from build123d import *

# Parameters (mm, degrees)
BOSS_EXTRUDE1_DEPTH = 12.7
FILLET2_R           = 2.54
SKETCH2_R           = 3.175
CUT_EXTRUDE1_DEPTH  = 12.7


with BuildPart() as part:
    # Sketch1 → Boss-Extrude1 (new body)
    with BuildSketch(Plane.XY):
        with BuildLine():
            ThreePointArc((31.750000111, -25.4), (6.35, -1.11e-07), (31.749999889, 25.4))
            Line((31.749999889, 25.4), (-63.5, 25.4))
            Line((-63.5, 25.4), (-63.5, -25.4))
            Line((-63.5, -25.4), (31.750000111, -25.4))
        make_face()
        with BuildLine():
            ThreePointArc((49.97081502, -7.62), (12, 0), (49.97081502, 7.62))
            Line((49.97081502, 7.62), (55.980055716, 7.62))
            ThreePointArc((55.980055716, 7.62), (46.776842604, 20.478134714), (31.749999889, 25.4))
            ThreePointArc((31.749999889, 25.4), (6.35, -1.11e-07), (31.750000111, -25.4))
            ThreePointArc((31.750000111, -25.4), (46.776842694, -20.478134648), (55.980055716, -7.62))
            Line((55.980055716, -7.62), (49.97081502, -7.62))
        make_face()
        with BuildLine():
            ThreePointArc((49.97081502, 7.62), (50.823284356, 5.125653506), (51.335987338, 2.54))
            Line((51.335987338, 2.54), (57.022680903, 2.54))
            ThreePointArc((57.022680903, 2.54), (56.631355132, 5.106678649), (55.980055716, 7.62))
            Line((55.980055716, 7.62), (49.97081502, 7.62))
        make_face()
        with BuildLine():
            ThreePointArc((55.980055716, 7.62), (56.631355132, 5.106678649), (57.022680903, 2.54))
            Line((57.022680903, 2.54), (63.5, 2.54))
            Line((63.5, 2.54), (63.5, 7.62))
            Line((63.5, 7.62), (55.980055716, 7.62))
        make_face()
        with BuildLine():
            Line((57.022680903, -2.54), (51.335987338, -2.54))
            ThreePointArc((51.335987338, -2.54), (50.823284356, -5.125653506), (49.97081502, -7.62))
            Line((49.97081502, -7.62), (55.980055716, -7.62))
            ThreePointArc((55.980055716, -7.62), (56.631355132, -5.106678649), (57.022680903, -2.54))
        make_face()
        with BuildLine():
            Line((63.5, -2.54), (57.022680903, -2.54))
            ThreePointArc((57.022680903, -2.54), (56.631355132, -5.106678649), (55.980055716, -7.62))
            Line((55.980055716, -7.62), (63.5, -7.62))
            Line((63.5, -7.62), (63.5, -2.54))
        make_face()
        with BuildLine():
            Line((63.5, -7.62), (55.980055716, -7.62))
            ThreePointArc((55.980055716, -7.62), (46.776842694, -20.478134648), (31.750000111, -25.4))
            Line((31.750000111, -25.4), (63.5, -25.4))
            Line((63.5, -25.4), (63.5, -7.62))
        make_face()
    extrude(amount=BOSS_EXTRUDE1_DEPTH)

    # Fillet2
    fillet2_edges = [part.edges().sort_by_distance(p)[0] for p in [
        (51.335987338, 2.54, 6.35),
        (51.335987338, -2.54, 6.35),
    ]]
    fillet(fillet2_edges, radius=FILLET2_R)

    # Sketch2 → Cut-Extrude1 (cut)
    with BuildSketch(Plane.XY.offset(12.7)):
        with Locations((-50.8, -9.525)):
            Circle(SKETCH2_R)
        with Locations((-41.819743879, -0.544743879)):
            Circle(SKETCH2_R)
        with Locations((-32.839487758, 8.435512242)):
            Circle(SKETCH2_R)
        with Locations((-41.148, -9.525)):
            Circle(SKETCH2_R)
        with Locations((-32.167743879, -0.544743879)):
            Circle(SKETCH2_R)
        with Locations((-23.187487758, 8.435512242)):
            Circle(SKETCH2_R)
        with Locations((-31.496, -9.525)):
            Circle(SKETCH2_R)
        with Locations((-22.515743879, -0.544743879)):
            Circle(SKETCH2_R)
        with Locations((-13.535487758, 8.435512242)):
            Circle(SKETCH2_R)
        with Locations((-21.844, -9.525)):
            Circle(SKETCH2_R)
        with Locations((-12.863743879, -0.544743879)):
            Circle(SKETCH2_R)
        with Locations((-3.883487758, 8.435512242)):
            Circle(SKETCH2_R)
    extrude(amount=-CUT_EXTRUDE1_DEPTH, mode=Mode.SUBTRACT)


solid = part.part
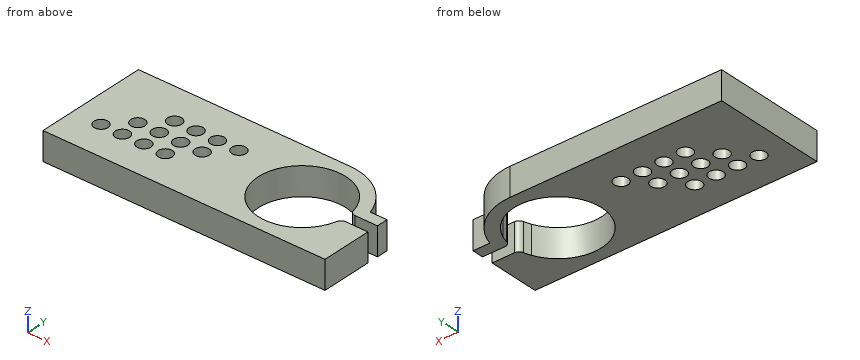
Build history of the part. All positions in model axes, mm. Give positions to 0.01 mm unless a question says otherwise; leave off trailing zeros. Write each loop counter-clockwise with the first axis right and the second up, starting at its lowest first coordinate (ties: lowest second). Pieces come first, ordered by that corner, then holes. Notation, with made-up numbers: (-5.5, 3.5) - (37.5, 3.5) arc R15 cw to (37.5, 9.5) - close; hole circle Ø10 at (78.25, 52). An arc over 180 degrees is marked (long way). Use one line per item in the form item = value. Start each with the question number.
1. Band-saw the part on B-B on y = 10. Write the cut outline in (x, z).
2. Band-saw the part on C-C on z = 10.75. Count the separate pieces of the cut face and the enclosed holes in it, plus the area to 3 significant figures.
3. Band-saw the part on D-D on x = -22.5. Write the cut outline in (y, z).
4. Probe line 1 (Y direction, x = 57, z = 10.5); line 2 (X direction, y = -7.5, z = 12); line 3 (X direction, y = 9, z = 4.5). List the from-to ranges inside material, lowest first. Write a range as [from, to].
5. Band-saw the part on A-A on x = -50.8. Write the cut outline in (y, z), plus the area to 3 significant figures.
6. Drop flat-ended pins along their axis: pin 1 Ø5 at (y, z) = (11.5, 8) entering from +X; pin 2 Ø4 at (x, z) = (60.5, 8) entering from +Y. Give the stop position or say it passes through.
Conclusion:
q1.outline = (-63.5, 0) - (-35.6, 0) - (-35.6, 12.7) - (-63.5, 12.7) - close; (-30.08, 0) - (-25.95, 0) - (-25.95, 12.7) - (-30.08, 12.7) - close; (-20.42, 0) - (-16.3, 0) - (-16.3, 12.7) - (-20.42, 12.7) - close; (-10.77, 0) - (-6.65, 0) - (-6.65, 12.7) - (-10.77, 12.7) - close; (-1.12, 0) - (14.72, 0) - (14.72, 12.7) - (-1.12, 12.7) - close; (48.78, 0) - (55.1, 0) - (55.1, 12.7) - (48.78, 12.7) - close
q2.separate_pieces = 1
q2.enclosed_holes = 12
q2.area = 4,530 mm²
q3.outline = (-25.4, 0) - (-12.63, 0) - (-12.63, 12.7) - (-25.4, 12.7) - close; (-6.42, 0) - (-3.72, 0) - (-3.72, 12.7) - (-6.42, 12.7) - close; (2.63, 0) - (5.34, 0) - (5.34, 12.7) - (2.63, 12.7) - close; (11.54, 0) - (25.4, 0) - (25.4, 12.7) - (11.54, 12.7) - close
q4.line_1 = [-25.4, -2.54], [2.54, 7.62]
q4.line_2 = [-63.5, -53.25], [-48.35, -43.59], [-38.7, -33.94], [-29.05, -24.29], [-19.4, 13.48], [50.02, 63.5]
q4.line_3 = [-63.5, -35.96], [-29.72, -26.31], [-20.06, -16.66], [-10.41, -7.01], [-0.76, 14.17], [49.33, 55.5]
q5.outline = (-25.4, 0) - (-12.7, 0) - (-12.7, 12.7) - (-25.4, 12.7) - close; (-6.35, 0) - (25.4, 0) - (25.4, 12.7) - (-6.35, 12.7) - close
q5.area = 565 mm²
q6.pin_1 = 55.5
q6.pin_2 = 7.62
